Geometry check sheet. Reference: the model listing, model coordinates, mm. A direction names the side the tool comes from. Give positions to 0.01 mm unless a question says otherwise; leave off trailing zeros. Write each loop counter-clockwise with the first axis right and the second up, starting at its lowest first coordinate (ties: lowest second). Pieces come first, ordered by that corner, then holes. Notation, with made-up numbers: M 28.5,-10.75 L 81.5,-10.75 A20 ccw 81.5,26.25 Z; hole C -28,57.5 d5. An arc over 180 degrees is marked long. One line per item, written item: value. Start each with the question number.
1. Cross-section at A-A on x = 165.1. Record the cut outline in (y, z), then the cut area to 3 significant figures.
2. Tool access check on faces 5 (the face through (227, 9, -139.7)), 6 (the face through (59, 9, -139.7)), 7 (the face through (137, 9, 0)). Record the directions out of +Z, -Z, +X, -X, +Y, -Y that give a thin tool (end or side, any length) a straight path to the whole face; none if there is none.
3. Release check for a two-part mould opening along X. For faces 1 (the face through (120.65, 10, -152)), 2 (the face through (159.466, 9.658, -149.47)), 3 (the face through (177.8, 10, -152)), 4 (the face through (137, 0, -84)) record: pulls with the +X half, pulls with the -X half, needs draft (parallel to the pull), parting line crosses it, or undercut.
4. Cross-section at D-D on x = 229. Record the cut outline in (y, z), then the cut area to 3 significant figures.
5. Gauge pin test, flat ends, axial feed: pin 1 (9.5 mm diameter, centred on y = 6.5, z = -157, fed in from -X); pin 2 (9.5 mm diameter, centred on x = 82, y = 11.5, fed in from -Z); pin 3 (11.5 mm diameter, centred on x = 165.1, z = -152.4, fed in from +Y). Record the tip position at first contact, or that the pin passes through.
6. Cross-section at B-B on z = -152.4. Record the cut outline in (x, y), then the cut area to 3 significant figures.
7. Scan lines: line 1 (X direction, y = 14.75, z = -152.4); line 2 (X direction, y = 15, z = -158); line 3 (Z direction, x = 240.5, y = 1). Record each from-to range of solid material in increasing order.
8. Cross-section at C-C on y = 3.5. Record the cut outline in (x, z), then the cut area to 3 significant figures.
from build123d import *

# Parameters (mm, degrees)
SKETCH1_W           = 277.876
SKETCH1_H           = 139.7
BOSS_EXTRUDE2_DEPTH = 19.05
SKETCH2_W           = 57.15
SKETCH2_H           = 25.4
SKETCH2_R           = 6.35
BOSS_EXTRUDE3_DEPTH = 19.05


with BuildPart() as part:
    # Sketch1 → Boss-Extrude2 (new body)
    with BuildSketch(Plane(origin=(0, 0, 0), x_dir=(1, 0, 0), z_dir=(0, 1, 0))):
        with Locations((138.938, 69.85)):
            Rectangle(SKETCH1_W, SKETCH1_H)
    extrude(amount=BOSS_EXTRUDE2_DEPTH)

    # Sketch2 → Boss-Extrude3 (add)
    with BuildSketch(Plane(origin=(0, 19.05, 0), x_dir=(1, 0, 0), z_dir=(0, 1, 0))):
        with Locations((149.225, 152.4)):
            Rectangle(SKETCH2_W, SKETCH2_H)
        with Locations(Location((133.35, 152.4, 0), (0, 0, 270))):
            Circle(SKETCH2_R, mode=Mode.SUBTRACT)
        with Locations(Location((165.1, 152.4, 0), (0, 0, 270))):
            Circle(SKETCH2_R, mode=Mode.SUBTRACT)
    extrude(amount=-BOSS_EXTRUDE3_DEPTH)


solid = part.part
Report:
1. outline: M 0,-165.1 L 19.05,-165.1 L 19.05,-158.75 L 0,-158.75 Z; M 0,-146.05 L 19.05,-146.05 L 19.05,0 L 0,0 Z
1. area: 2,900 mm^2
2. face 5: -Z, +X, +Y, -Y
2. face 6: -Z, -X, +Y, -Y
2. face 7: +Z, +X, -X, +Y, -Y
3. face 1: pulls with the -X half
3. face 2: undercut
3. face 3: pulls with the +X half
3. face 4: needs draft
4. outline: M 0,-139.7 L 19.05,-139.7 L 19.05,0 L 0,0 Z
4. area: 2,660 mm^2
5. pin 1: stops at x = 120.65
5. pin 2: stops at z = -139.7
5. pin 3: passes through
6. outline: M 120.65,0 L 127,0 L 127,19.05 L 120.65,19.05 Z; M 139.7,0 L 158.75,0 L 158.75,19.05 L 139.7,19.05 Z; M 171.45,0 L 177.8,0 L 177.8,19.05 L 171.45,19.05 Z
6. area: 605 mm^2
7. line 1: x = 120.65 to 127, 139.7 to 158.75, 171.45 to 177.8
7. line 2: x = 120.65 to 130.36, 136.34 to 162.11, 168.09 to 177.8
7. line 3: z = -139.7 to 0
8. outline: M 0,-139.7 L 120.65,-139.7 L 120.65,-165.1 L 177.8,-165.1 L 177.8,-139.7 L 277.88,-139.7 L 277.88,0 L 0,0 Z; hole C 133.35,-152.4 d12.7; hole C 165.1,-152.4 d12.7
8. area: 40,000 mm^2
